from build123d import *

# Parameters (mm, degrees)
F0_R     = 5.5626
F1_DEPTH = 25.4


with BuildPart() as f1:
    # F0 (on Top) → F1 (new body)
    with BuildSketch(Plane.XY):
        with BuildLine():
            Line((78.160428, 63.5), (0, 63.5))
            Line((0, 63.5), (0, 0))
            Line((0, 0), (78.160428, 0))
            ThreePointArc((78.160428, 0), (69.525671, 4.28997), (66.04, 13.279572))
            Line((66.04, 13.279572), (66.04, 51.379572))
            ThreePointArc((66.04, 51.379572), (69.589991, 59.950009), (78.160428, 63.5))
        make_face()
        with BuildLine():
            ThreePointArc((84.098042, 61.946005), (81.229229, 63.105067), (78.160428, 63.5))
            ThreePointArc((78.160428, 63.5), (69.589991, 59.950009), (66.04, 51.379572))
            Line((66.04, 51.379572), (66.04, 13.279572))
            ThreePointArc((66.04, 13.279572), (69.525671, 4.28997), (78.160428, 0))
            ThreePointArc((78.160428, 0), (82.159702, 0.238573), (85.907615, 1.654291))
            Line((85.907615, 1.654291), (118.946738, 20.220023))
            ThreePointArc((118.946738, 20.220023), (125.4252, 31.29172), (118.946738, 42.363416))
            Line((118.946738, 42.363416), (84.098042, 61.946005))
        make_face()
        with Locations((79.375, 13.279572)):
            Circle(F0_R, mode=Mode.SUBTRACT)
        with Locations((112.7252, 31.29172)):
            Circle(F0_R, mode=Mode.SUBTRACT)
        with Locations((78.160428, 51.379572)):
            Circle(F0_R, mode=Mode.SUBTRACT)
    extrude(amount=F1_DEPTH)


solid = f1.part
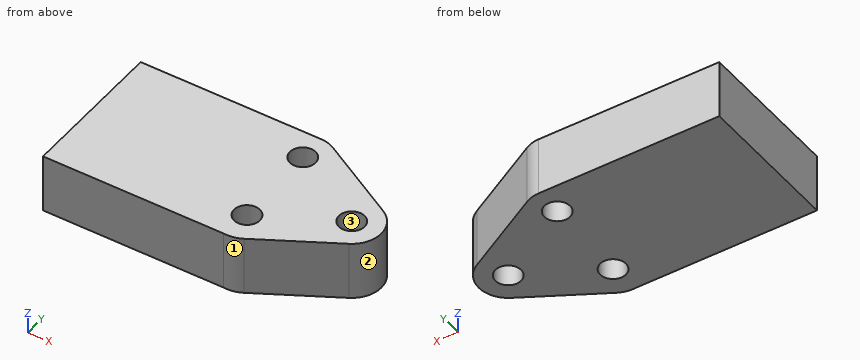
Check sheet for the modelled part. Datum: model origin and axes. Units: mm. Face numbers are marked on the shaded views. Coordinates: 2 decimals unless noted, no trailing zeros. Write each loop counter-clockwise with the first axis right and the second up, starting at its lowest first coordinate (ties: lowest second). Pieces come first, ordered by that corner, then holes.
Item 1: Depth check by flat-ended pin: pin 1 Ø8 at (y, z) = (36.5, 6) entering from +X; pin 2 Ø6.5 at (x, y) = (112.73, 31.29) entering from +Z; pin 3 Ø10 at (x, z) = (93, 14) entering from -Y. Enter the tip coordinate at first touch or a pass-through.
Numbers:
pin 1: stops at x = 125.37
pin 2: passes through
pin 3: stops at y = 2.83
Item 2: Cross-section at A-A on y = 53.5. Record the boundary of the cut face in (x, z).
Numbers:
outline: (0, 0) - (73.02, 0) - (73.02, 25.4) - (0, 25.4) - close; (83.3, 0) - (99.13, 0) - (99.13, 25.4) - (83.3, 25.4) - close
Item 3: Scan lines: probe 1 along Y at (x, z) = (63.5, 14.5); probe 2 along X at (y, z) = (47, 9.75); probe 3 along X at (y, z) = (10, 21.5). Record each from-to range of solid material in increasing order.
Numbers:
probe 1: y = 0 to 63.5
probe 2: x = 0 to 74.73, 81.59 to 110.7
probe 3: x = 0 to 74.88, 83.87 to 100.76
Item 4: Cross-section at C-C on x = 81. Record the boundary of the cut face in (y, z), then the cut area to 3 significant figures.
Numbers:
outline: (0.04, 0) - (7.96, 0) - (7.96, 25.4) - (0.04, 25.4) - close; (18.6, 0) - (46.6, 0) - (46.6, 25.4) - (18.6, 25.4) - close; (56.16, 0) - (63.16, 0) - (63.16, 25.4) - (56.16, 25.4) - close
area: 1,090 mm2
Item 5: Cross-section at D-D on y = 9. Record the boundary of the cut face in (x, z).
Numbers:
outline: (0, 0) - (75.82, 0) - (75.82, 25.4) - (0, 25.4) - close; (82.93, 0) - (98.98, 0) - (98.98, 25.4) - (82.93, 25.4) - close
Item 6: Cross-section at B-B on z = 21. Record the boundary of the cut face in (x, y) (3 decimals).
Numbers:
outline: (0, 0) - (78.16, 0) arc R13.335 ccw to (85.908, 1.654) - (118.947, 20.22) arc R12.7 ccw to (118.947, 42.363) - (84.098, 61.946) arc R12.12 ccw to (78.16, 63.5) - (0, 63.5) - close; hole circle Ø11.125 at (78.16, 51.38); hole circle Ø11.125 at (79.375, 13.28); hole circle Ø11.125 at (112.725, 31.292)
Item 7: Mould release check, pull along Y, two halves, no side actions. Record for the marked faces 1, 2 and 3: released by +Y, released by -Y, zero draft, split by the parting line, or undercut.
Numbers:
face 1: released by -Y
face 2: split by the parting line
face 3: undercut
